```python
from build123d import *

# Parameters (mm, degrees)
F1_DEPTH = 21
F2_W     = 12.5
F2_H     = 20
F2_W_2   = 24
F3_DEPTH = 20
F5_DEPTH = 0.5
F6_R     = 7
F7_DEPTH = 25


with BuildPart() as f1:
    # F0 (on Front) → F1 (new body)
    with BuildSketch(Plane.XZ):
        Polygon((0, 12), (0, 0), (24, 0), (24, 12), (36, 12), (36, 36), (24, 36), (24, 53), (0, 53), (0, 36), (-12, 36), (-12, 12), align=None)
    extrude(amount=F1_DEPTH)

    # F2 (on face) → F3 (join)
    with BuildSketch(Plane.XY.offset(53)):
        with Locations((30.25, -10.5)):
            Rectangle(F2_W, F2_H)
        with Locations((12, -10.5)):
            Rectangle(F2_W_2, F2_H)
        with Locations((-6.25, -10.5)):
            Rectangle(F2_W, F2_H)
    extrude(amount=F3_DEPTH)

    # F4 (on face) → F5 (join)
    with BuildSketch(Plane(origin=(0, -0.5, 0), x_dir=(-1, 0, 0), z_dir=(0, 1, 0))):
        Polygon((12.5, 73), (-36.5, 73), (-36.5, 53), (-24, 53), (0, 53), (12.5, 53), align=None)
    extrude(amount=F5_DEPTH)

    # F6 (on face) → F7 (cut)
    with BuildSketch(Plane(origin=(0, 0, 0), x_dir=(-1, 0, 0), z_dir=(0, 1, 0))):
        with Locations((-12, 63)):
            Circle(F6_R)
    extrude(amount=-F7_DEPTH, mode=Mode.SUBTRACT)


solid = f1.part
```
Model file for the job. Use its own axes, mm. A direction names the side the tool comes from. Coordinates: 2 decimals unless noted, no trailing zeros. Loops run counter-clockwise (first coordinate to the right, second up) from the corner with the lowest first, then second, coordinate; pieces in that order, holes last. Notation, with made-up numbers: M 23,-32 L 63,-32 A14 ccw 63,-17 Z; hole C 12.25,62.25 d5. An arc over 180 degrees is marked long. Use CSV: the item, a comma, the result in double quotes. Start each with the question number.
1. Band-saw the part on C-C, the plane x = 33.5. List the corners of the cut face in (y, z), then the cut area to 3 significant figures.
2. Flat gauge pins, fed straight in: pin 1 (1.5 mm diameter, centred on x = 3.5, y = -5.5, fed in from -Z); pin 2 (3.5 mm diameter, centred on y = -15.5, z = 8, fed in from -X); pin 3 (6 mm diameter, centred on x = -9, y = -7.5, fed in from -Z); pin 4 (11 mm diameter, centred on x = 12, z = 63, fed in from -Y). Where does each tip first touch, or does it go through?
3. Band-saw the part on A-A, the plane y = -10. List the corners of the cut face in (x, z), then the cut area to 3 significant figures.
4. Band-saw the part on D-D, the plane x = 12. List the corners of the cut face in (y, z).
5. Band-saw the part on B-B, the plane z = 63. List the corners of the cut face in (x, y), then the cut area to 4 significant figures.
6. Probe probe 1 along Z at (x, y) = (12, -8); probe 2 along Z at (x, y) = (-8.5, -3.25); probe 3 along X at (y, z) = (-8.5, 17.5). List the from-to ranges inside material, lowest first. Write a range as [from, to].
7. Two-plate mould, pull along Z, no slides. Class faces 1 (the flat face through (-6, -10, 36)), 2 (the flat face through (-6, -10, 12)), 3 (the flat face through (0, -10, 6)): pulls with the +Z half, pulls with the -Z half, needs draft (parallel to the pull), parting line crosses it, or undercut.
8. Tool access for faces 4 (the flat face through (6, -20.5, 58)), 5 (the flat face through (36, -10, 24)), 6 (the flat face through (30, -10, 53)), 7 (the flat face through (-12, -10, 24)): list every direction of +Z, -Z, +X, -X, +Y, -Y with a clear straight run to the whole face (end or side of a thin tool).
Entries:
1,outline,"M -21,12 L 0,12 L 0,36 L -21,36 Z; M -20.5,53 L 0,53 L 0,73 L -20.5,73 Z"
1,area,"914 mm2"
2,pin 1,"stops at z = 0"
2,pin 2,"stops at x = 0"
2,pin 3,"stops at z = 12"
2,pin 4,"passes through"
3,outline,"M -12.5,53 L 0,53 L 0,36 L -12,36 L -12,12 L 0,12 L 0,0 L 24,0 L 24,12 L 36,12 L 36,36 L 24,36 L 24,53 L 36.5,53 L 36.5,73 L -12.5,73 Z; hole C 12,63 d14"
3,area,"2,670 mm2"
4,outline,"M -21,0 L 0,0 L 0,56 L -20.5,56 L -20.5,53 L -21,53 Z; M -20.5,70 L 0,70 L 0,73 L -20.5,73 Z"
5,outline,"M -12.5,-20.5 L 5,-20.5 L 5,0 L -12.5,0 Z; M 19,-20.5 L 36.5,-20.5 L 36.5,0 L 19,0 Z"
5,area,"717.5 mm2"
6,probe 1,"z = [0, 56], [70, 73]"
6,probe 2,"z = [12, 36], [53, 73]"
6,probe 3,"x = [-12, 36]"
7,face 1,"undercut"
7,face 2,"pulls with the -Z half"
7,face 3,"needs draft"
8,face 4,"+Z, +X, -X, -Y"
8,face 5,"-Z, +X, +Y, -Y"
8,face 6,"+X, +Y, -Y"
8,face 7,"-Z, -X, +Y, -Y"
